Autodesk Inventor part; units mm, degrees
ref_plane "YZ Plane" through (0, 0, 0) normal (1, 0, 0) x (0, 1, 0)
ref_plane "XZ Plane" through (0, 0, 0) normal (0, 1, 0) x (-1, 0, 0)
ref_plane "XY Plane" through (0, 0, 0) normal (0, 0, 1) x (1, 0, 0)
sketch "Sketch1" plane through (0, 0, 0) normal (0, 0, 1) x (1, 0, 0)
  line L0 (0, 0) -> (50.8, 0)
  line L1 (50.8, 0) -> (50.8, 50.8)
  line L2 (50.8, 50.8) -> (0, 50.8)
  line L3 (0, 50.8) -> (0, 0)
  line L4 (6.35, 6.35) -> (44.45, 6.35)
  line L5 (44.45, 6.35) -> (44.45, 44.45)
  line L6 (44.45, 44.45) -> (6.35, 44.45)
  line L7 (6.35, 44.45) -> (6.35, 6.35)
  dimension "d0" = 50.8
  dimension "d1" = 50.8
  dimension "d2" = 6.35
extrude "Extrusion1" add sketch "Sketch1" along normal blind 246.8
sketch "Sketch2" plane through (0, 0, 0) normal (0, -1, 0) x (1, 0, 0)
  circle A0 centre (25.4, 149.2) radius 4
  circle A1 centre (25.4, 199.2) radius 4
  line L0 (0, 246.8) -> (50.8, 246.8)
  line L1 (0, 0) -> (50.8, 0)
  point P0 (25.4, 246.8)
  dimension "d5" = 8
  dimension "d6" = 8
  dimension "d7" = 50
  dimension "d8" = 149.2
extrude "Extrusion2" cut sketch "Sketch2" against normal through all
properties part number "ST22" material "Aluminum 6061"
Build history of the part. All positions in model axes, mm. A direction names the side the tool comes from. Round coordinates to 2 decimals unless told otherwise and drop trailing zeros. Loops run counter-clockwise (first coordinate to the right, second up) from the corner with the lowest first, then second, coordinate; pieces in that order, holes last.
Item 1: Saw through at A-A (z = 149.2). List the corners of the cut face in (x, y), then the cut area to 3 significant figures.
Item 2: Two-plate mould, pull along Z, no slides. Class faces 1 (the face through (24.533, 47.581, 145.295)), 2 (the face through (24.533, 47.581, 195.295)), 3 (the face through (25, 0, 122)), 4 (the face through (48, 26, 0)): released by +Z, released by -Z, zero draft, split by the parting line, or undercut.
Item 3: Saw through at C-C (z = 88). List the corners of the cut face in (x, y).
Item 4: Drill centre lines: line 1 along Z through (x, y) = (25.4, 2); line 2 along X through (y, z) = (29.5, 159). Where is each one in solid material? Low to high.
Item 5: Saw through at B-B (x = 25.4). List the corners of the cut face in (y, z), then the cut area to 3 significant figures.
Item 6: Which spindle directions (+Z, -Z, +X, -X, +Y, -Y) get a long thin tool onto all of the face, cutting with end or side? Do faces 5 (the face through (26, 44.45, 122)), 6 (the face through (24.533, 3.131, 195.295)). Say none if no direction does.
Worked answers:
1. outline: (0, 0) - (21.4, 0) - (21.4, 6.35) - (6.35, 6.35) - (6.35, 44.45) - (21.4, 44.45) - (21.4, 50.8) - (0, 50.8) - close; (29.4, 0) - (50.8, 0) - (50.8, 50.8) - (29.4, 50.8) - (29.4, 44.45) - (44.45, 44.45) - (44.45, 6.35) - (29.4, 6.35) - close
1. area: 1,030 mm2
2. face 1: undercut
2. face 2: undercut
2. face 3: zero draft
2. face 4: released by -Z
3. outline: (0, 0) - (50.8, 0) - (50.8, 50.8) - (0, 50.8) - close; hole (6.35, 6.35) - (44.45, 6.35) - (44.45, 44.45) - (6.35, 44.45) - close
4. line 1: z = 0 to 145.2, 153.2 to 195.2, 203.2 to 246.8
4. line 2: x = 0 to 6.35, 44.45 to 50.8
5. outline: (0, 0) - (6.35, 0) - (6.35, 145.2) - (0, 145.2) - close; (0, 153.2) - (6.35, 153.2) - (6.35, 195.2) - (0, 195.2) - close; (0, 203.2) - (6.35, 203.2) - (6.35, 246.8) - (0, 246.8) - close; (44.45, 0) - (50.8, 0) - (50.8, 145.2) - (44.45, 145.2) - close; (44.45, 153.2) - (50.8, 153.2) - (50.8, 195.2) - (44.45, 195.2) - close; (44.45, 203.2) - (50.8, 203.2) - (50.8, 246.8) - (44.45, 246.8) - close
5. area: 2,930 mm2
6. face 5: +Z, -Z
6. face 6: +Y, -Y
